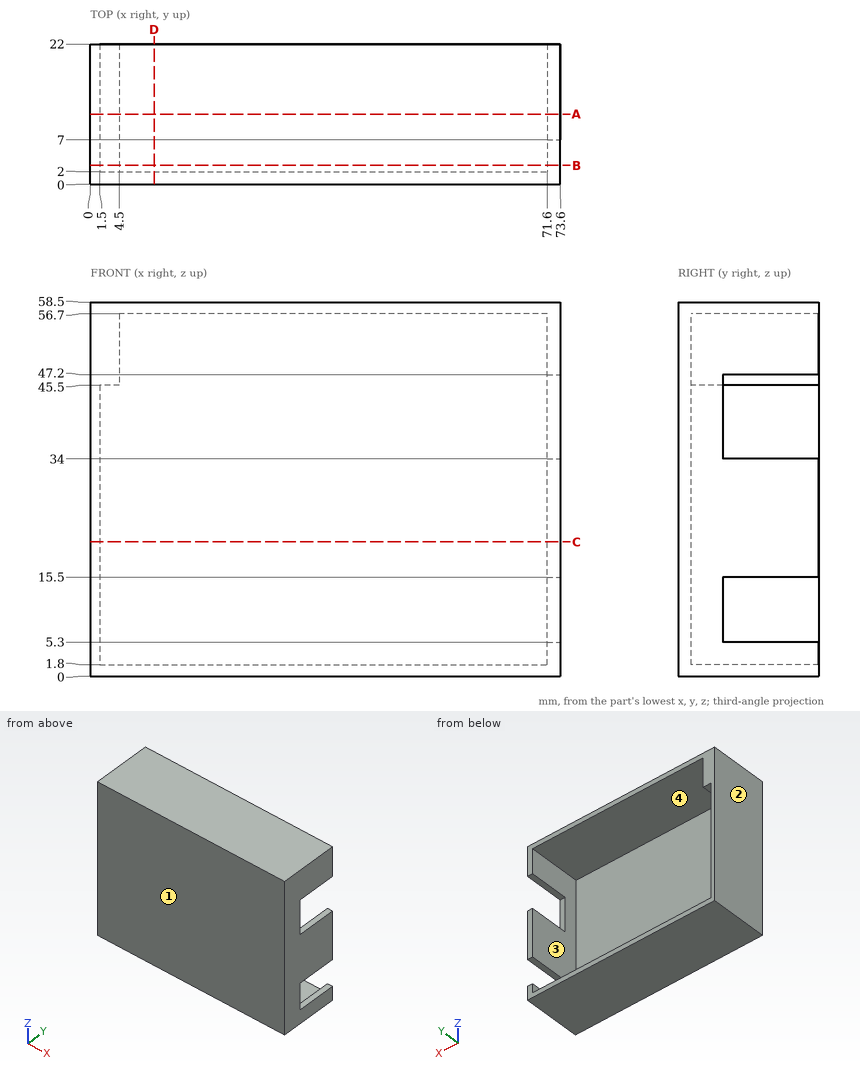
Geometry check sheet. Reference: drawing and pictorial views, mm from the part's lowest x, y, z. Give positions to 0.01 mm unless a question says otherwise; leave off trailing zeros. Write each loop counter-clockwise with the first axis right and the second up, starting at its lowest first coordinate (ties: lowest second). Pieces come first, ordered by that corner, then holes. Notation, with made-up numbers: M 70,86.5 L 113,86.5 A21 ccw 113,119.5 Z; hole C 60.25,-7 d8. An arc over 180 degrees is marked long. Answer as CSV lines item,"result". Start each with the question number.
Q1. Release check for a two-part mould opening along X. For the marked faces 1, 2, 3 and 4 record: pulls with the +X half, pulls with the -X half, needs draft (parallel to the pull), parting line crosses it, or undercut.
Q2. Section check B-B, the plane y = 3. Record the cut outline in (x, z).
Q3. Go/stop test with flat-tipped pins: pin 1 (1 mm diameter, centred on x = 73, z = 12, fed in from +Y); pin 2 (6 mm diameter, centred on x = 20.5, z = 36.5, fed in from +Y); pin 3 (1 mm diameter, centred on y = 8, z = 44.5, fed in from +X). Record where each tip stops, or that it passes through.
Q4. Section check D-D, the plane x = 10. Record the cut outline in (y, z).
Q5. Section check C-C, the plane z = 21. Record the cut outline in (x, y).
Q6. Section check A-A, the plane y = 11. Record the cut outline in (x, z), then the cut area to 3 significant figures.
Q7. Material ranges on L1, parallel to X at y = 8.5, z = 21; L2, parallel to Z at x = 54.5, y = 2.75; L3, parallel to X at y = 14.25, z = 49, recorded low to high.
Geometry says:
1,face 1,"needs draft"
1,face 2,"pulls with the -X half"
1,face 3,"undercut"
1,face 4,"undercut"
2,outline,"M 0,0 L 73.6,0 L 73.6,58.5 L 0,58.5 Z; hole M 1.5,1.8 L 71.6,1.8 L 71.6,56.7 L 4.5,56.7 L 4.5,45.5 L 1.5,45.5 Z"
3,pin 1,"y = 7"
3,pin 2,"y = 2"
3,pin 3,"x = 1.5"
4,outline,"M 0,0 L 22,0 L 22,1.8 L 2,1.8 L 2,56.7 L 22,56.7 L 22,58.5 L 0,58.5 Z"
5,outline,"M 0,0 L 73.6,0 L 73.6,22 L 71.6,22 L 71.6,2 L 1.5,2 L 1.5,22 L 0,22 Z"
6,outline,"M 0,0 L 73.6,0 L 73.6,5.3 L 71.6,5.3 L 71.6,1.8 L 1.5,1.8 L 1.5,45.5 L 4.5,45.5 L 4.5,56.7 L 71.6,56.7 L 71.6,47.2 L 73.6,47.2 L 73.6,58.5 L 0,58.5 Z; M 71.6,15.5 L 73.6,15.5 L 73.6,34 L 71.6,34 Z"
6,area,"444 mm^2"
7,L1,"0 to 1.5, 71.6 to 73.6"
7,L2,"0 to 1.8, 56.7 to 58.5"
7,L3,"0 to 4.5, 71.6 to 73.6"
